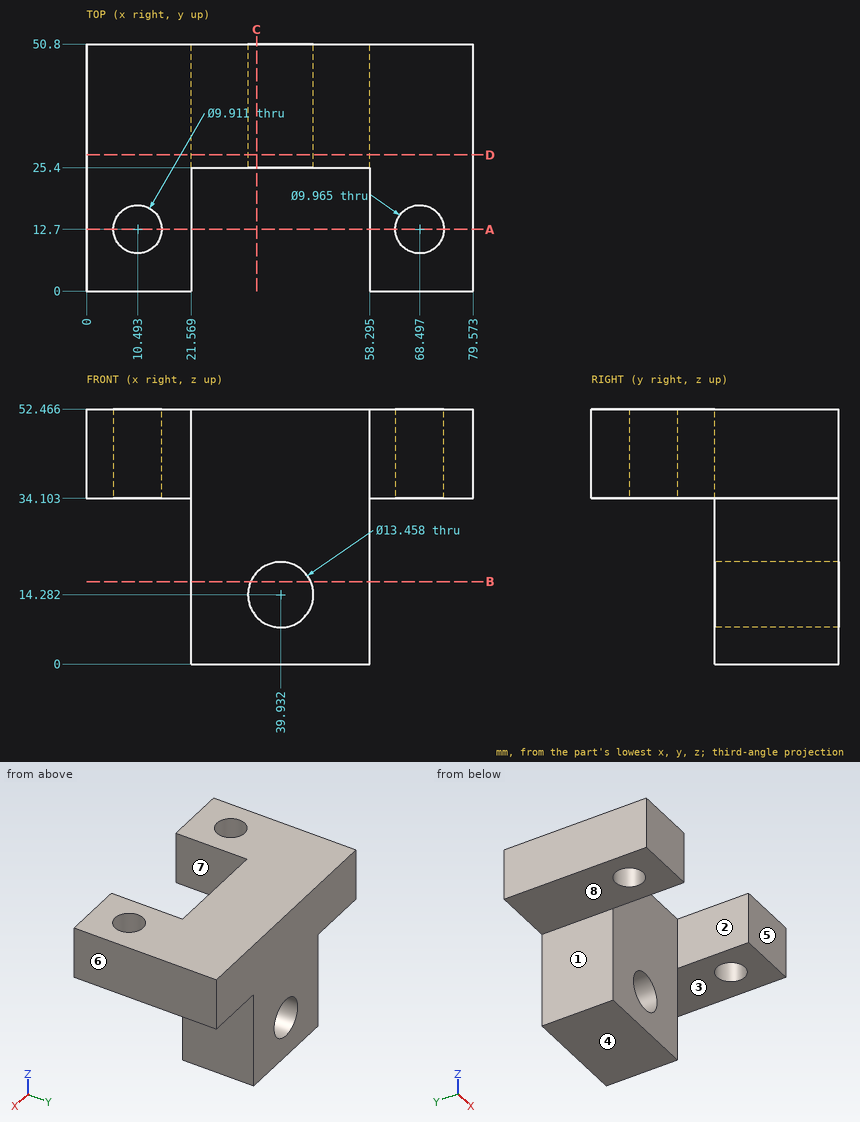
Here's the drawing with two shaded views (mm, measured from the low corner). I have some questions. A direction names the side the tool comes from. Give positions to 0.01 mm unless a question says otherwise; leave off trailing zeros. Loops run counter-clockwise (first coordinate to the right, second up) from the corner with the lowest first, then second, coordinate; pieces in that order, holes last. Notation, with made-up numbers: M 44,21.25 L 81,21.25 A30 cw 81,53.25 Z; hole C -32,-28.75 d6. An arc over 180 degrees is marked long. Use one line per item in the form item = value. Start each with the question number.
Q1. If we section it at A-A (y = 12.7): Write out the boundary of the cut face in (x, z) (1 decimal).
Q2. Which directions (+Z, -Z, +X, -X, +Y, -Y) give clear straight access to the entire face, cutting with the end or side of a thin tool? Please do the marked faces 1, 2, 3, 4 and 5.
Q3. Will these pins go through, and if not, where does the flat tip stop? pin 1 Ø17 at (x, y) = (66.5, 17.5) entering from -Z; pin 2 Ø5 at (x, z) = (63, 31) entering from -Y; pin 3 Ø11 at (x, z) = (35.5, 34.5) entering from -Y; pin 4 Ø10 at (y, z) = (36.5, 6) entering from -X.
Q4. I need wall thicknesses on line 1 along X through (y, z) = (12.7, 46.75) (1 decimal); line 2 along Y through (x, z) = (56.5, 16.5); line 3 along Z through (x, y) = (19.5, 39) (1 decimal). Which ranges of each line are inside material? Lowest first, please.
Q5. Thinking about a two-plate mould opening in X: for the marked faces 6, 7 and 8, which applies, +X half, -X half, draft (parallel to the pull), parting line (faces both ways), or undercut?
Q6. If we section it at C-C (x = 35): Write out the boundary of the cut face in (y, z) (1 decimal).
Q7. If we section it at D-D (y = 28): Write out the boundary of the cut face in (x, z) (1 decimal).
Q8. If we section it at B-B (z = 17): Write out the boundary of the cut face in (x, y) (1 decimal), then the cut area to 3 significant figures.
Taken from the geometry:
q1.outline = M 0,34.1 L 5.5,34.1 L 5.5,52.5 L 0,52.5 Z; M 15.4,34.1 L 21.6,34.1 L 21.6,52.5 L 15.4,52.5 Z; M 58.3,34.1 L 63.5,34.1 L 63.5,52.5 L 58.3,52.5 Z; M 73.5,34.1 L 79.6,34.1 L 79.6,52.5 L 73.5,52.5 Z
q2.face_1 = -Z, -X, +Y, -Y
q2.face_2 = +Z, -Z, -Y
q2.face_3 = -Z, +X, +Y, -Y
q2.face_4 = -Z, +X, -X, +Y, -Y
q2.face_5 = +Z, -Z, +X, -X, -Y
q3.pin_1 = 34.1
q3.pin_2 = through
q3.pin_3 = 25.4
q3.pin_4 = 21.57
q4.line_1 = 0 to 5.5, 15.4 to 21.6, 58.3 to 63.5, 73.5 to 79.6
q4.line_2 = 25.4 to 50.8
q4.line_3 = 34.1 to 52.5
q5.face_6 = +X half
q5.face_7 = undercut
q5.face_8 = draft
q6.outline = M 25.4,0 L 50.8,0 L 50.8,9.7 L 25.4,9.7 Z; M 25.4,18.9 L 50.8,18.9 L 50.8,52.5 L 25.4,52.5 Z
q7.outline = M 0,34.1 L 21.6,34.1 L 21.6,0 L 58.3,0 L 58.3,34.1 L 79.6,34.1 L 79.6,52.5 L 0,52.5 Z; hole C 39.9,14.3 d13.5
q8.outline = M 21.6,25.4 L 33.8,25.4 L 33.8,50.8 L 21.6,50.8 Z; M 46.1,25.4 L 58.3,25.4 L 58.3,50.8 L 46.1,50.8 Z
q8.area = 620 mm^2
